Check sheet for the drawn part. Datum: minimum x, y, z corner. Units: mm. Round coordinates to 2 decimals unless told otherwise and drop trailing zeros. Order: outer loops, then holes, each group sorted by start corner. A loop starts at its lowest first (then second) coordinate and runs counter-clockwise, first axis right, second up.
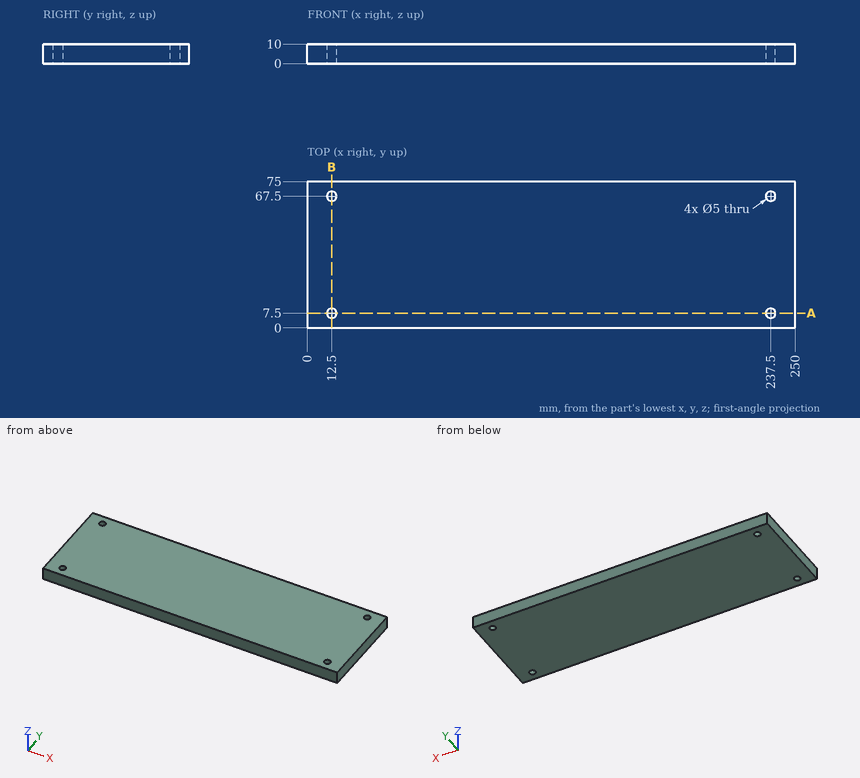
(1) Sectioned sample at B-B, the plane x = 12.5. Record the cut outline in (y, z).
Returned:
outline: (0, 0) - (5, 0) - (5, 10) - (0, 10) - close; (10, 0) - (65, 0) - (65, 10) - (10, 10) - close; (70, 0) - (75, 0) - (75, 10) - (70, 10) - close
(2) Material ranges on line 1 (Y direction, x = 12.5, z = 2.75); line 2 (X direction, y = 8, z = 5), recorded low to high.
Returned:
line 1: y = 0 to 5, 10 to 65, 70 to 75
line 2: x = 0 to 10.05, 14.95 to 235.05, 239.95 to 250
(3) Sectioned sample at A-A, the plane y = 7.5. Record the cut outline in (x, z), and give its area (3 significant figures).
Returned:
outline: (0, 0) - (10, 0) - (10, 10) - (0, 10) - close; (15, 0) - (235, 0) - (235, 10) - (15, 10) - close; (240, 0) - (250, 0) - (250, 10) - (240, 10) - close
area: 2,400 mm2
